Part model, mm, in its own coordinate system. Face numbers are marked on the shaded views. A direction names the side the tool comes from. Give positions to 0.01 mm unless a question says otherwise; leave off trailing zeros. Order: outer loops, then holes, each group sorted by start corner. A loop starts at its lowest first (then second) coordinate and runs counter-clockwise, first axis right, second up. Notation, with made-up numbers: M 60,-14.75 L 103,-14.75 A26 ccw 103,16.25 Z; hole C -14.5,67.5 d5. An arc over 180 degrees is marked long. Return JSON: item names as keys, results as strings.
from build123d import *

# Parameters (mm, degrees)
EXTRUDE_1_DEPTH          = 30
SHELL_1_T                = -3
CUT_EXTRUDE_1_REACH      = 72.356
SKETCH_3_R               = 3
SKETCH_4_W               = 45
SKETCH_4_H               = 45
SKETCH_4_W_2             = 42.3
SKETCH_4_H_2             = 42.3
EXTRUDE_3_DEPTH          = 20
SKETCH_11_R              = 1.5
CUT_EXTRUDE_4_DEPTH      = 70.130311731
SKETCH_7_W               = 2
SKETCH_7_H               = 19.5
EXTRUDE_5_DEPTH          = 20
PATTERN_CIRCULAR_1_COUNT = 2
PATTERN_CIRCULAR_1_ANGLE = 90
SKETCH_10_R              = 5
CUT_EXTRUDE_3_DEPTH      = 71.356236397
FILLET_1_R               = 5
EXTRUDE_START            = -2.5
EXTRUDE_6_DEPTH          = 2.5


with BuildPart() as part:
    # 草图1 → 凸台-拉伸1 (new body)
    with BuildSketch(Plane.XY):
        with BuildLine():
            Line((-35, 45), (35, 45))
            ThreePointArc((35, 45), (42.071067812, 42.071067812), (45, 35))
            Line((45, 35), (45, -35))
            ThreePointArc((45, -35), (42.071067812, -42.071067812), (35, -45))
            Line((35, -45), (-35, -45))
            ThreePointArc((-35, -45), (-42.071067812, -42.071067812), (-45, -35))
            Line((-45, -35), (-45, 35))
            ThreePointArc((-45, 35), (-42.071067812, 42.071067812), (-35, 45))
        make_face()
    extrude(amount=EXTRUDE_1_DEPTH)

    # 抽壳1
    shell_1_openings = [part.faces().sort_by_distance(p)[0] for p in [
        (0, 0, 30),
    ]]
    offset(amount=SHELL_1_T, openings=shell_1_openings, kind=Kind.INTERSECTION)

    # 草图3 → 切除-拉伸1 (cut, up to next)
    with BuildSketch(Plane.XY.offset(30), mode=Mode.PRIVATE) as cut_extrude_1_sk1:
        with Locations((-34, 34)):
            Circle(SKETCH_3_R)
    cut_extrude_1_tool1 = extrude(cut_extrude_1_sk1.sketch, amount=-CUT_EXTRUDE_1_REACH, mode=Mode.PRIVATE) & part.part
    # 草图3 → 切除-拉伸1 (cut, up to next)
    with BuildSketch(Plane.XY.offset(30), mode=Mode.PRIVATE) as cut_extrude_1_sk2:
        with Locations((34, 34)):
            Circle(SKETCH_3_R)
    cut_extrude_1_tool2 = extrude(cut_extrude_1_sk2.sketch, amount=-CUT_EXTRUDE_1_REACH, mode=Mode.PRIVATE) & part.part
    # 草图3 → 切除-拉伸1 (cut, up to next)
    with BuildSketch(Plane.XY.offset(30), mode=Mode.PRIVATE) as cut_extrude_1_sk3:
        with Locations((34, -34)):
            Circle(SKETCH_3_R)
    cut_extrude_1_tool3 = extrude(cut_extrude_1_sk3.sketch, amount=-CUT_EXTRUDE_1_REACH, mode=Mode.PRIVATE) & part.part
    # 草图3 → 切除-拉伸1 (cut, up to next)
    with BuildSketch(Plane.XY.offset(30), mode=Mode.PRIVATE) as cut_extrude_1_sk4:
        with Locations((-34, -34)):
            Circle(SKETCH_3_R)
    cut_extrude_1_tool4 = extrude(cut_extrude_1_sk4.sketch, amount=-CUT_EXTRUDE_1_REACH, mode=Mode.PRIVATE) & part.part
    add(cut_extrude_1_tool1.solids().sort_by_distance((-34, 34, 30))[0], mode=Mode.SUBTRACT)
    add(cut_extrude_1_tool2.solids().sort_by_distance((34, 34, 30))[0], mode=Mode.SUBTRACT)
    add(cut_extrude_1_tool3.solids().sort_by_distance((34, -34, 30))[0], mode=Mode.SUBTRACT)
    add(cut_extrude_1_tool4.solids().sort_by_distance((-34, -34, 30))[0], mode=Mode.SUBTRACT)

    # 草图4 → 凸台-拉伸3 (add)
    with BuildSketch(Plane.XY.offset(3)):
        Rectangle(SKETCH_4_W, SKETCH_4_H)
        Rectangle(SKETCH_4_W_2, SKETCH_4_H_2, mode=Mode.SUBTRACT)
    extrude(amount=EXTRUDE_3_DEPTH)

    # 草图11 → 切除-拉伸4 (cut, through all)
    with BuildSketch(Plane.XY.offset(3)):
        with Locations((-15.5, -15.5)):
            Circle(SKETCH_11_R)
        with Locations((15.5, -15.5)):
            Circle(SKETCH_11_R)
        with Locations((15.5, 15.5)):
            Circle(SKETCH_11_R)
        with Locations((-15.5, 15.5)):
            Circle(SKETCH_11_R)
    extrude(amount=-CUT_EXTRUDE_4_DEPTH, mode=Mode.SUBTRACT)

    # 草图7 → 凸台-拉伸5 (add)
    with BuildSketch(Plane.XY.offset(3)):
        with Locations((0, 32.25)):
            Rectangle(SKETCH_7_W, SKETCH_7_H)
        with Locations((0, -32.25)):
            Rectangle(SKETCH_7_W, SKETCH_7_H)
    extrude_5 = extrude(amount=EXTRUDE_5_DEPTH)

    # 阵列(圆周)1: 凸台-拉伸5 ×2 about axis
    pattern_circular_1_axis = Axis((0, 0, -2), (0, 0, 1))
    for i in range(1, PATTERN_CIRCULAR_1_COUNT):
        add(extrude_5.rotate(pattern_circular_1_axis, i * PATTERN_CIRCULAR_1_ANGLE / (PATTERN_CIRCULAR_1_COUNT - 1)))

    # 草图10 → 切除-拉伸3 (cut, through all)
    with BuildSketch(Plane(origin=(0, 0, 0), x_dir=(-1, 0, 0), z_dir=(0, 0, -1))):
        Circle(SKETCH_10_R)
    extrude(amount=-CUT_EXTRUDE_3_DEPTH, mode=Mode.SUBTRACT)

    # 圆角1
    fillet_1_edges = [part.edges().sort_by_distance(p)[0] for p in [
        (0, 42, 23),
        (0, -42, 23),
        (-42, 0, 23),
        (42, 0, 23),
    ]]
    fillet(fillet_1_edges, radius=FILLET_1_R)

    # 草图12 → 凸台-拉伸6 (add)
    with BuildSketch(Plane.XY.offset(30).offset(EXTRUDE_START)):
        with BuildLine():
            Line((34, 42), (35, 42))
            ThreePointArc((35, 42), (39.949747468, 39.949747468), (42, 35))
            Line((42, 35), (42, 34))
            Line((42, 34), (54, 34))
            ThreePointArc((54, 34), (57.535533906, 35.464466094), (59, 39))
            Line((59, 39), (59, 54))
            ThreePointArc((59, 54), (57.535533906, 57.535533906), (54, 59))
            Line((54, 59), (39, 59))
            ThreePointArc((39, 59), (35.464466094, 57.535533906), (34, 54))
            Line((34, 54), (34, 42))
        make_face()
        with BuildLine():
            Line((42, -34), (54, -34))
            ThreePointArc((54, -34), (57.535533906, -35.464466094), (59, -39))
            Line((59, -39), (59, -54))
            ThreePointArc((59, -54), (57.535533906, -57.535533906), (54, -59))
            Line((54, -59), (39, -59))
            ThreePointArc((39, -59), (35.464466094, -57.535533906), (34, -54))
            Line((34, -54), (34, -42))
            Line((34, -42), (35, -42))
            ThreePointArc((35, -42), (39.949747468, -39.949747468), (42, -35))
            Line((42, -35), (42, -34))
        make_face()
        with BuildLine():
            Line((-42, -35), (-42, -34))
            Line((-42, -34), (-54, -34))
            ThreePointArc((-54, -34), (-57.535533906, -35.464466094), (-59, -39))
            Line((-59, -39), (-59, -54))
            ThreePointArc((-59, -54), (-57.535533906, -57.535533906), (-54, -59))
            Line((-54, -59), (-39, -59))
            ThreePointArc((-39, -59), (-35.464466094, -57.535533906), (-34, -54))
            Line((-34, -54), (-34, -42))
            Line((-34, -42), (-35, -42))
            ThreePointArc((-35, -42), (-39.949747468, -39.949747468), (-42, -35))
        make_face()
        with BuildLine():
            Line((-42, 35), (-42, 34))
            Line((-42, 34), (-54, 34))
            ThreePointArc((-54, 34), (-57.535533906, 35.464466094), (-59, 39))
            Line((-59, 39), (-59, 54))
            ThreePointArc((-59, 54), (-57.535533906, 57.535533906), (-54, 59))
            Line((-54, 59), (-39, 59))
            ThreePointArc((-39, 59), (-35.464466094, 57.535533906), (-34, 54))
            Line((-34, 54), (-34, 42))
            Line((-34, 42), (-35, 42))
            ThreePointArc((-35, 42), (-39.949747468, 39.949747468), (-42, 35))
        make_face()
    extrude(amount=EXTRUDE_6_DEPTH)


solid = part.part
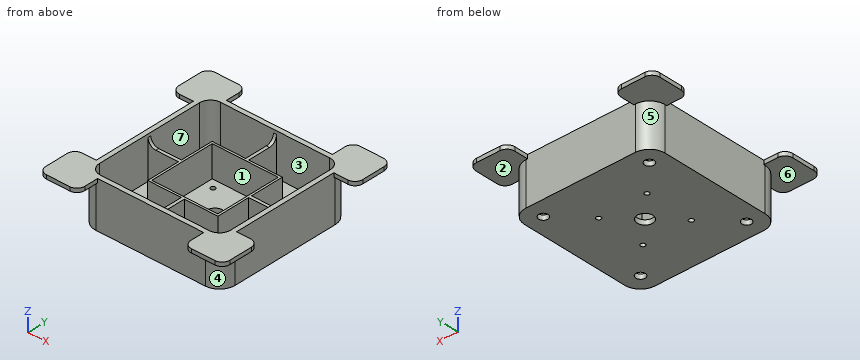
Q1. Band-saw the part on D-D (y = 8). Give the cut face in (x, z), then the cut area to 3 significant figures.
Established:
{"outline": "M -45,0 L 45,0 L 45,30 L 42,30 L 42,3 L 22.5,3 L 22.5,23 L 21.15,23 L 21.15,3 L -21.15,3 L -21.15,23 L -22.5,23 L -22.5,3 L -42,3 L -42,30 L -45,30 Z", "area": "486 mm²"}
Q2. Band-saw the part on B-B (x = 15.5). Give the cut face in (y, z).
Established:
{"outline": "M -45,0 L -17,0 L -17,3 L -21.15,3 L -21.15,23 L -22.5,23 L -22.5,3 L -42,3 L -42,30 L -45,30 Z; M -14,0 L 14,0 L 14,3 L -14,3 Z; M 17,0 L 45,0 L 45,30 L 42,30 L 42,3 L 22.5,3 L 22.5,23 L 21.15,23 L 21.15,3 L 17,3 Z"}
Q3. Two-plate mould, pull along X, no slides. Class the marked faces 1, 2, 3 and 4: +X half, -X half, draft (parallel to the pull), parting line (faces both ways), or undercut.
Established:
{"face 1": "undercut", "face 2": "draft", "face 3": "undercut", "face 4": "+X half"}
Q4. Pin check, flat tips, straight feed: pin 1 (15.5 mm diameter, centred on x = -28.5, z = 10.5, fed in from -Y); pin 2 (2 mm diameter, centred on x = 13, y = 26.5, fed in from -Z); pin 3 (12 mm diameter, centred on x = -8, y = 26, fed in from +Z); pin 4 (16 mm diameter, centred on y = -7.5, z = 12, fed in from +X). Stop position of each tip, or through.
Established:
{"pin 1": "stops at y = -45", "pin 2": "stops at z = 0", "pin 3": "stops at z = 23", "pin 4": "stops at x = 45"}
Q5. 3-axis set-ups, long thin cutter, end or side, ignore diameter. For the marked faces 5, 6 and 7: which of +Z, -Z, +X, -X, +Y, -Y reach the whole face in a straight line?
Established:
{"face 5": "-Z, -X, +Y", "face 6": "-Z, -X, -Y", "face 7": "+Z"}
Q6. Probe line 1 along Y through (x, z) = (15.5, 1.05); line 2 along X through (y, z) = (-12, 10); line 3 along Y through (x, z) = (34, 8.75). List the from-to ranges inside material, lowest first.
Established:
{"line 1": "y = -45 to -17, -14 to 14, 17 to 45", "line 2": "x = -45 to -42, -22.5 to -21.15, 21.15 to 22.5, 42 to 45", "line 3": "y = -45 to -42, -1 to 1, 42 to 45"}
Q7. Band-saw the part on A-A (y = 51). Give the cut face in (x, z), then the cut area to 3 significant figures.
Established:
{"outline": "M -59,27.5 L -34,27.5 L -34,30 L -59,30 Z; M 34,27.5 L 59,27.5 L 59,30 L 34,30 Z", "area": "125 mm²"}
